from build123d import *

# Parameters (mm, degrees)
F1_DEPTH = 25
F2_R     = 50
F3_DEPTH = 25


with BuildPart() as f1:
    # F0 (on Top) → F1 (new body)
    with BuildSketch(Plane.XY):
        with BuildLine():
            Line((500, -500), (500, 0))
            ThreePointArc((500, 0), (-353.553391, 353.553391), (0, -500))
            Line((0, -500), (500, -500))
        make_face()
    extrude(amount=F1_DEPTH)

    # F2 (on face) → F3 (cut, through all)
    with BuildSketch(Plane.XY.offset(25)):
        with BuildLine():
            ThreePointArc((-229.809704, 229.809704), (-218.971066, 246.030871), (-215.165043, 265.165043))
            ThreePointArc((-215.165043, 265.165043), (-311.35902, 284.299215), (-229.809704, 229.809704))
        make_face()
        with Locations((265.165043, -265.165043)):
            Circle(F2_R)
    extrude(amount=-F3_DEPTH, mode=Mode.SUBTRACT)


solid = f1.part
Check sheet for the modelled part. Datum: model origin and axes. Units: mm. Round coordinates to 2 decimals unless told otherwise and drop trailing zeros. Loops run counter-clockwise (first coordinate to the right, second up) from the corner with the lowest first, then second, coordinate; pieces in that order, holes last. Notation, with made-up numbers: (11.25, -7.75) - (51.25, -7.75) arc R12 cw to (51.25, 13.25) - close; hole circle Ø10 at (14.5, 43.5). An arc over 180 degrees is marked (long way). Answer as CSV lines item,"result". Start each with the question number.
Item 1: Section check B-B (z = 15.75). Record the boundary of the cut face in (x, y), and give its area (3 significant figures).
Item 2: Depth check by flat-ended pin: P1, Ø12, axis at y = 197.5, z = 5, coming from the -X side. Enter the tip coordinate at first touch or a pass-through.
Item 3: Section check C-C (x = -266.5). Record the boundary of the cut face in (y, z), and give its area (3 significant figures).
Item 4: Scan lines: line 1 (Y direction, x = -270, z = 11); line 2 (Y direction, x = -223, z = 6.25); line 3 (X direction, y = -386, z = 10). Record each from-to range of solid material in increasing order. Write a range as [from, to].
Item 5: Section check A-A (x = 283.5). Record the boundary of the cut face in (y, z), and give its area (3 significant figures).
Item 6: Release check for a two-part mould opening along X. For faces 1 (the cylindrical face through (292.04, -223, 12.68)), 2 (the flat face through (-7, 7, 0)), 3 (the cylindrical face through (-341.7, 365.02, 12.32)) record: +X half, -X half, draft (parallel to the pull), parting line (faces both ways), or undercut.
Item 7: Section check D-D (y = 104.5). Record the boundary of the cut face in (x, z).
Report:
1,outline,"(0, -500) - (500, -500) - (500, 0) arc R500 ccw (long way) to start; hole (-229.81, 229.81) arc R50 ccw to (-215.17, 265.17) arc R50 ccw (long way) to start; hole circle Ø100 at (265.17, -265.17)"
1,area,"823,000 mm2"
2,P1,"stops at x = -461.87"
3,outline,"(-423.06, 0) - (215.18, 0) - (215.18, 25) - (-423.06, 25) - close; (315.15, 0) - (423.06, 0) - (423.06, 25) - (315.15, 25) - close"
3,area,"18,700 mm2"
4,line 1,"y = [-420.83, 215.4], [314.93, 420.83]"
4,line 2,"y = [-447.52, 238.29], [292.04, 447.52]"
4,line 3,"x = [-317.81, 500]"
5,outline,"(-500, 0) - (-311.68, 0) - (-311.68, 25) - (-500, 25) - close; (-218.65, 0) - (411.86, 0) - (411.86, 25) - (-218.65, 25) - close"
5,area,"20,500 mm2"
6,face 1,"undercut"
6,face 2,"draft"
6,face 3,"parting line"
7,outline,"(-488.96, 0) - (488.96, 0) - (488.96, 25) - (-488.96, 25) - close"
